Autodesk Fusion 360 part; units mm, degrees
sketch "Sketch1" plane through (0, 0, 0) normal (0, 1, 0) x (1, 0, 0)
  circle A0 centre (0, 0) radius 30
  dimension "d1" = 60
extrude "Extrude1" add sketch "Sketch1" along normal blind 300
ref_plane "WorkPlane2" through (0, 0, 30) normal (0, 0, 1) x (1, 0, 0)
sketch "Sketch5" plane through (0, 0, 30) normal (0, 0, 1) x (1, 0, 0)
  circle A0 centre (0, 63) radius 10
  dimension "d16" = 63
  dimension "d17" = 20
extrude "Extrude5" cut sketch "Sketch5" against normal blind 10
pattern_circular "C-Pattern2" count 4 over 360 about axis through (0, 1.75, 0) along (0, 1, 0) of "Extrude5"
thread "Thread1"
thread "Thread2"
thread "Thread3"
thread "Thread4"
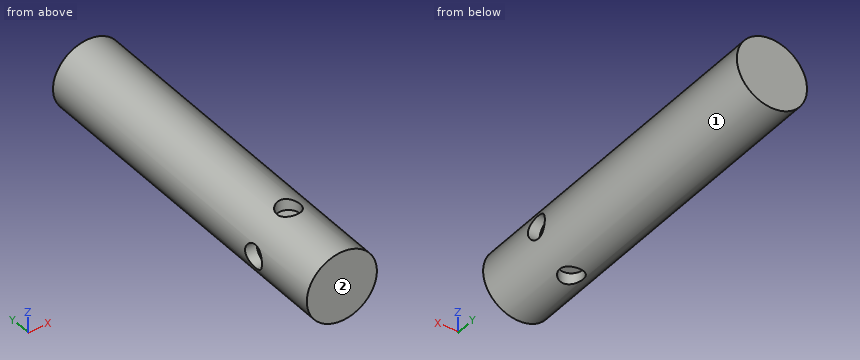
CAD build for the part. Positions are in the model's coordinates, mm. Face numbers are marked on the shaded views. Give positions to 0.01 mm unless a question says otherwise; leave off trailing zeros. Loops run counter-clockwise (first coordinate to the right, second up) from the corner with the lowest first, then second, coordinate; pieces in that order, holes last. Notation, with made-up numbers: M 50,1 L 72,1 A22 ccw 72,18 Z; hole C 2,65 d6. An arc over 180 degrees is marked long. Answer in a Markdown table with one row per item. Add a question column.
Item 1: Band-saw the part on A-A on z = 0. Give the cut face in (x, y).
Item 2: Drop flat-ended pins along their axis: P1, Ø12, axis at x = 0, y = 63, coming from the -Z side; P2, Ø2, axis at x = -8.5, y = 170.5, coming from the -Z side; P3, Ø1.5, axis at y = 250, z = -2.5, coming from the +X side; P4, Ø3, axis at x = -22.5, z = -22, coming from the +Y side. Give the stop position or say it passes through.
Item 3: Band-saw the part on D-D on y = 126.5. Give the cut face in (x, z).
Item 4: Band-saw the part on C-C on y = 63. Give the cut face in (x, z), then the cut area to 3 significant figures.
Item 5: Mould opens along X. For the marked faces 1 and 2 say: +X half, -X half, draft (parallel to the pull), parting line (faces both ways), or undercut.
Item 6: Probe probe 1 along Y at (x, z) = (0, 25.75); probe 2 along Z at (x, y) = (1.5, 27); probe 3 along X at (y, z) = (63, 27). List the from-to ranges inside material, lowest first.
Item 7: Band-saw the part on B-B on x = 0. Give the cut face in (y, z), then the cut area to 3 significant figures.
Reply:
| question | item | result |
|---|---|---|
| 1 | outline | M -30,0 L 30,0 L 30,53 L 20,53 L 20,73 L 30,73 L 30,300 L -30,300 L -30,73 L -20,73 L -20,53 L -30,53 Z |
| 2 | P1 | stops at z = -20 |
| 2 | P2 | stops at z = -29.05 |
| 2 | P3 | stops at x = 29.95 |
| 2 | P4 | stops at y = 300 |
| 3 | outline | C 0,0 d60 |
| 4 | outline | M -28.28,-10 A30 ccw -10,-28.28 L -10,-20 L 10,-20 L 10,-28.28 A30 ccw 28.28,-10 L 20,-10 L 20,10 L 28.28,10 A30 ccw 10,28.28 L 10,20 L -10,20 L -10,28.28 A30 ccw -28.28,10 L -20,10 L -20,-10 Z |
| 4 | area | 2,070 mm^2 |
| 5 | face 1 | parting line |
| 5 | face 2 | draft |
| 6 | probe 1 | y = 0 to 53, 73 to 300 |
| 6 | probe 2 | z = -29.96 to 29.96 |
| 6 | probe 3 | x = -13.08 to -10, 10 to 13.08 |
| 7 | outline | M 0,-30 L 53,-30 L 53,-20 L 73,-20 L 73,-30 L 300,-30 L 300,30 L 73,30 L 73,20 L 53,20 L 53,30 L 0,30 Z |
| 7 | area | 17,600 mm^2 |
